```python
from build123d import *

# Parameters (mm, degrees)
F0_W     = 80
F0_H     = 60
F1_DEPTH = 40
F2_R     = 5
F3_SIZE  = 2
F4_T     = -4
F5_R     = 7.5
F6_DEPTH = 40.001
F7_W     = 47.272053
F7_H     = 29.239059
F8_DEPTH = 20.1
F9_R     = 5


with BuildPart() as f1:
    # F0 (on Top) → F1 (new body)
    with BuildSketch(Plane.XY):
        with Locations((40, 30)):
            Rectangle(F0_W, F0_H)
    extrude(amount=F1_DEPTH)

    # F2
    f2_edges = [f1.edges().sort_by_distance(p)[0] for p in [
        (80, 60, 20),
        (80, 0, 20),
        (0, 0, 20),
        (0, 60, 20),
    ]]
    fillet(f2_edges, radius=F2_R)

    # F3
    f3_edges = [f1.edges().sort_by_distance(p)[0] for p in [
        (40, 0, 40),
    ]]
    chamfer(f3_edges, length=F3_SIZE)

    # F4
    f4_openings = [f1.faces().sort_by_distance(p)[0] for p in [
        (40, 30, 0),
    ]]
    offset(amount=F4_T, openings=f4_openings)

    # F5 (on face) → F6 (cut, through all)
    with BuildSketch(Plane.XY.offset(40)):
        with Locations((20, 15)):
            Circle(F5_R)
    extrude(amount=-F6_DEPTH, mode=Mode.SUBTRACT)

    # F7 (on face) → F8 (cut)
    with BuildSketch(Plane.XZ):
        with Locations((71.118602, 33.85017)):
            Rectangle(F7_W, F7_H)
    extrude(amount=-F8_DEPTH, mode=Mode.SUBTRACT)

    # F9
    f9_edges = [f1.edges().sort_by_distance(p)[0] for p in [
        (47.482576, 2, 19.230641),
        (47.482576, 20.1, 38),
        (78, 20.1, 19.230641),
    ]]
    fillet(f9_edges, radius=F9_R)


solid = f1.part
```
Read the model definition and answer for the solid it produces. Units are mm, in the model's axes. A direction names the side the tool comes from. Round coordinates to 2 decimals unless told otherwise and drop trailing zeros. Write each loop counter-clockwise with the first axis right and the second up, starting at its lowest first coordinate (ties: lowest second). Pieces come first, ordered by that corner, then holes. Notation, with made-up numbers: M -9,29 L 2,29 A16 ccw 2,33 Z; hole C -22,52.5 d3. An arc over 180 degrees is marked long. One line per item, written item: value.
Q1. Find section D-D on z = 34. Write down the section's boundary in (x, y), plus the area to 3 significant figures.
Data:
outline: M 0,5 A5 ccw 5,0 L 47.48,0 L 47.48,4 L 5,4 A1 cw 4,5 L 4,55 A1 cw 5,56 L 75,56 A1 cw 76,55 L 76,20.1 L 80,20.1 L 80,55 A5 ccw 75,60 L 5,60 A5 ccw 0,55 Z
area: 846 mm2
Q2. Flat-ended cylindrical pins translate along their axes: pin 1 Ø19.5 at (x, y) = (20, 15) entering from -Z; pin 2 Ø12 at (y, z) = (8.5, 34) entering from +X; pin 3 Ø12.5 at (x, z) = (69.5, 29.5) entering from -Y. Find the tip coordinate at first contact, or state that the pin passes through.
Data:
pin 1: z = 36
pin 2: x = 47.48
pin 3: y = 55.66
Q3. Find section B-B on z = 12. Write down the section's boundary in (x, y).
Data:
outline: M 0,5 A5 ccw 5,0 L 75,0 A5 ccw 80,5 L 80,55 A5 ccw 75,60 L 5,60 A5 ccw 0,55 Z; hole M 4,5 A1 ccw 5,4 L 75,4 A1 ccw 76,5 L 76,55 A1 ccw 75,56 L 5,56 A1 ccw 4,55 Z
Q4. Find section A-A on x = 61.5. Write down the section's boundary in (y, z).
Data:
outline: M 0,0 L 4,0 L 4,19.23 L 0,19.23 Z; M 20.1,36 L 56,36 L 56,0 L 60,0 L 60,38 L 58,40 L 20.1,40 Z
Q5. Find section C-C on y = 21.5. Write down the section's boundary in (x, z), plus the area to 3 significant figures.
Data:
outline: M 0,0 L 4,0 L 4,36 L 16.26,36 L 16.26,40 L 2,40 L 0,38 Z; M 23.74,36 L 76,36 L 76,0 L 80,0 L 80,38 L 78,40 L 23.74,40 Z
area: 574 mm2
Q6. Straight lines are drawn through the part: line 1 (Y direction, x = 33, z = 21); line 2 (X direction, y = 9.5, z = 16); line 3 (Z direction, x = 18.5, y = 29.5). For each, find the intervals that lie inside material, in ascending order. Write a range as [from, to].
Data:
line 1: [0, 4], [56, 60]
line 2: [0, 4], [76, 80]
line 3: [36, 40]
Q7. For a pull along Y with two mould halves and no side action, classify faces 1 (the flat face through (39, 36, 36)), 2 (the flat face through (79, 37, 39)), 3 (the cylindrical face through (1, 58, 19)) as +Y half, -Y half, draft (parallel to the pull), parting line (faces both ways), or undercut.
Data:
face 1: undercut
face 2: draft
face 3: +Y half
Q8. Which of the six approach directions +Z, -Z, +X, -X, +Y, -Y give full straight-line access (tool end or side, diameter ignored) to faces 4 (the flat face through (4, 30, 18)), 5 (the cylindrical face through (48.986, 2.028, 20.656)), 6 (the conical face through (77.71, 57.65, 39.21))?
Data:
face 4: -Z
face 5: +Z, +X, -Y
face 6: +Z, +X, +Y
